Can you work these out from the model? Positions are in its coordinate system, mm. A direction names the side the tool comes from. Round coordinates to 2 decimals unless told otherwise and drop trailing zeros. Loops run counter-clockwise (first coordinate to the right, second up) from the corner with the lowest first, then second, coordinate; pieces in that order, holes last. Notation, with made-up numbers: (-18.75, -17) -> (-11.75, -17) arc R25 ccw to (-11.75, 19) -> close; hole circle Ø9 at (76, 87.25). An arc over 180 degrees is marked (long way). Write item = value, one per line.
from build123d import *

# Parameters (mm, degrees)
BOSS_EXTRUDE1_DEPTH            = 20
BOSS_EXTRUDE2_DEPTH            = 15
F_1_0MM_DOWEL_HOLE1_AT_2_COUNT = 2
F_1_0MM_DOWEL_HOLE1_AT_2_PITCH = 31.941060089
F_1_0MM_DOWEL_HOLE1_AT_3_COUNT = 2
F_1_0MM_DOWEL_HOLE1_AT_3_PITCH = 29.907615952


with BuildPart() as part:
    # Sketch1 → Boss-Extrude1 (new, symmetric)
    with BuildSketch(Plane.XY):
        with BuildLine():
            Line((-23.598593643, 12.5), (-23.598593643, 5))
            Line((-23.598593643, 5), (-8.598593643, 5))
            Line((-8.598593643, 5), (-8.598593643, 12.5))
            Line((-8.598593643, 12.5), (1.401406357, 12.5))
            ThreePointArc((1.401406357, 12.5), (10.240241122, 16.161165235), (13.901406357, 25))
            Line((13.901406357, 25), (8.901406357, 25))
            ThreePointArc((8.901406357, 25), (1.401406357, 17.5), (-6.098593643, 25))
            Line((-6.098593643, 25), (-26.098593643, 25))
            ThreePointArc((-26.098593643, 25), (-33.598593643, 17.5), (-41.098593643, 25))
            Line((-41.098593643, 25), (-46.098593643, 25))
            ThreePointArc((-46.098593643, 25), (-42.437428408, 16.161165235), (-33.598593643, 12.5))
            Line((-33.598593643, 12.5), (-23.598593643, 12.5))
        make_face()
    extrude(amount=BOSS_EXTRUDE1_DEPTH, both=True)

    # Sketch1<3> → Boss-Extrude2 (add, symmetric)
    with BuildSketch(Plane.XY):
        with BuildLine():
            Line((-8.598593643, 12.5), (-8.598593643, 5))
            Line((-8.598593643, 5), (6.401406357, 5))
            Line((6.401406357, 5), (1.401406357, 0))
            Line((1.401406357, 0), (23.901406357, 0))
            Line((23.901406357, 0), (23.901406357, 15))
            Line((23.901406357, 15), (18.901406357, 15))
            Line((18.901406357, 15), (18.901406357, 25))
            Line((18.901406357, 25), (13.901406357, 25))
            ThreePointArc((13.901406357, 25), (10.240241122, 16.161165235), (1.401406357, 12.5))
            Line((1.401406357, 12.5), (-8.598593643, 12.5))
        make_face()
        with BuildLine():
            Line((-56.098593643, 15), (-56.098593643, 0))
            Line((-56.098593643, 0), (-33.598593643, 0))
            Line((-33.598593643, 0), (-38.598593643, 5))
            Line((-38.598593643, 5), (-23.598593643, 5))
            Line((-23.598593643, 5), (-23.598593643, 12.5))
            Line((-23.598593643, 12.5), (-33.598593643, 12.5))
            ThreePointArc((-33.598593643, 12.5), (-42.437428408, 16.161165235), (-46.098593643, 25))
            Line((-46.098593643, 25), (-51.098593643, 25))
            Line((-51.098593643, 25), (-51.098593643, 15))
            Line((-51.098593643, 15), (-56.098593643, 15))
        make_face()
    extrude(amount=BOSS_EXTRUDE2_DEPTH, both=True)

    # Sketch4 → Ø1.0mm Dowel Hole1 (revolve, cut)
    with BuildSketch(Plane(origin=(-17.146642207, 25, -15), x_dir=(0, 0, 1), z_dir=(1, 0, 0))):
        Polygon((0, 0), (0, 16.299038106), (2.25, 15), (2.25, 0), align=None)
    f_1_0mm_dowel_hole1 = revolve(axis=Axis((-17.146642207, 31.35, -15), (0, -1, 0)), mode=Mode.SUBTRACT)

    # Ø1.0mm Dowel Hole1 at 2: Ø1.0mm Dowel Hole1 ×2
    with Locations(*[Vector(0.9720418945746677, 0, 0.23480748538258048) * (i * F_1_0MM_DOWEL_HOLE1_AT_2_PITCH) for i in range(1, F_1_0MM_DOWEL_HOLE1_AT_2_COUNT)]):
        add(f_1_0mm_dowel_hole1, mode=Mode.SUBTRACT)

    # Ø1.0mm Dowel Hole1 at 3: Ø1.0mm Dowel Hole1 ×2
    with Locations(*[Vector(-0.9680461151483998, 0, 0.25077224516698626) * (i * F_1_0MM_DOWEL_HOLE1_AT_3_PITCH) for i in range(1, F_1_0MM_DOWEL_HOLE1_AT_3_COUNT)]):
        add(f_1_0mm_dowel_hole1, mode=Mode.SUBTRACT)

    # Mirror1: Ø1.0mm Dowel Hole1 across plane
    add(f_1_0mm_dowel_hole1.mirror(Plane.XY), mode=Mode.SUBTRACT)

    # Mirror1 copy 1 sketch → Mirror1 copy 1 (revolve, cut)
    with BuildSketch(Plane(origin=(13.901406357, 25, 7.5), x_dir=(0, 0, -1), z_dir=(1, 0, 0))):
        Polygon((0, 0), (0, -16.299038106), (2.25, -15), (2.25, 0), align=None)
    revolve(axis=Axis((13.901406357, 31.35, 7.5), (0, 1, 0)), mode=Mode.SUBTRACT)

    # Mirror1 copy 2 sketch → Mirror1 copy 2 (revolve, cut)
    with BuildSketch(Plane(origin=(-46.098593643, 25, 7.5), x_dir=(0, 0, -1), z_dir=(1, 0, 0))):
        Polygon((0, 0), (0, -16.299038106), (2.25, -15), (2.25, 0), align=None)
    revolve(axis=Axis((-46.098593643, 31.35, 7.5), (0, 1, 0)), mode=Mode.SUBTRACT)


solid = part.part
1. Suppose I cut it at C-C, the plane y = 16. List the corners of the cut face in (x, z) for me, and give its area (3 significant figures).
Entries:
outline = (-51.1, -15) -> (-42.27, -15) -> (-42.27, -20) -> (10.08, -20) -> (10.08, -15) -> (18.9, -15) -> (18.9, 15) -> (10.08, 15) -> (10.08, 20) -> (-42.27, 20) -> (-42.27, 15) -> (-51.1, 15) -> close; hole circle Ø4.5 at (-46.1, -7.5); hole circle Ø4.5 at (-46.1, 7.5); hole circle Ø4.5 at (-17.15, -15); hole circle Ø4.5 at (-17.15, 15); hole circle Ø4.5 at (13.9, -7.5); hole circle Ø4.5 at (13.9, 7.5)
area = 2,530 mm²
2. Suppose I cut it at B-B, the plane z = 3. List the corners of the cut face in (x, y) for me.
Entries:
outline = (-56.1, 0) -> (-33.6, 0) -> (-38.6, 5) -> (6.4, 5) -> (1.4, 0) -> (23.9, 0) -> (23.9, 15) -> (18.9, 15) -> (18.9, 25) -> (8.9, 25) arc R7.5 cw to (-6.1, 25) -> (-26.1, 25) arc R7.5 cw to (-41.1, 25) -> (-51.1, 25) -> (-51.1, 15) -> (-56.1, 15) -> close
3. I need wall thicknesses on line 1 (X direction, y = 13.5, z = 7.5); line 2 (X direction, y = 17.25, z = -7.5); line 3 (Z direction, x = -44.5, y = 19.5). Which ranges of each line are inside material? Lowest first, please. Write a range as [from, to].
Entries:
line_1 = [-56.1, -48.35], [-43.85, 11.65], [16.15, 23.9]
line_2 = [-51.1, -48.35], [-43.85, 11.65], [16.15, 18.9]
line_3 = [-20, -9.08], [-5.92, 5.92], [9.08, 20]
4. We'd pull the mould along Z, two halves only. Please class faces 1 (the flat face through (-44, 10, -15)), 2 (the flat face through (-44, 10, 15)), 3 (the cylindrical face through (-45.24, 17.6, -5.42)), 4 (the flat face through (-8.599, 9, -17)): released by +Z, released by -Z, zero draft, split by the parting line, or undercut.
Entries:
face_1 = released by -Z
face_2 = released by +Z
face_3 = undercut
face_4 = zero draft
5. For faces 5 (the cylindrical face through (-42.534, 16.259, -17.465)), 6 (the cylindrical face through (10.14, 16.06, 17.54)), 7 (the cylindrical face through (10.14, 16.06, -17.46)), 8 (the cylindrical face through (11.67, 17.6, -7.79)), which set-ups out of +Z, -Z, +X, -X, +Y, -Y let a thin tool reach every point of the face, with its end or its side?
Entries:
face_5 = -Z, -X, -Y
face_6 = +Z, +X, -Y
face_7 = -Z, +X, -Y
face_8 = +Y
6. Suppose I cut it at A-A, the plane y = 22.5. Count the separate pieces of the cut face and the enclosed holes in it, and give its area (3 significant figures).
Entries:
separate_pieces = 3
enclosed_holes = 6
area = 1,470 mm²
7. Suppose I cut it at D-D, the plane x = -3.5. List the corners of the cut face in (y, z) for me, and give its area (3 significant figures).
Entries:
outline = (5, -15) -> (12.5, -15) -> (12.5, -20) -> (19.32, -20) -> (19.32, 20) -> (12.5, 20) -> (12.5, 15) -> (5, 15) -> close
area = 498 mm²
8. I'm going to push flat-ended pins straight in: pin 1 (3 mm diameter, centred on y = 18, z = 7, fed in from -X); pin 2 (3 mm diameter, centred on x = -8.5, z = 1.5, fed in from -Y); pin 3 (12.5 mm diameter, centred on x = 11.5, y = 9, fed in from -Z). Where does each tip first touch, or does it pass through?
Entries:
pin_1 = -51.1
pin_2 = 5
pin_3 = -15
